Autodesk Inventor part; units mm, degrees
ref_plane "YZ Plane" through (0, 0, 0) normal (1, 0, 0) x (0, 1, 0)
ref_plane "XZ Plane" through (0, 0, 0) normal (0, 1, 0) x (-1, 0, 0)
ref_plane "XY Plane" through (0, 0, 0) normal (0, 0, 1) x (1, 0, 0)
sketch "スケッチ1" plane through (0, 0, 0) normal (1, 0, 0) x (0, 1, 0)
  circle A0 centre (0, 0) radius 19.5
  dimension "d0" = 39
extrude "押し出し1" add sketch "スケッチ1" along normal blind 3
sketch "スケッチ2" plane through (0, 0, 0) normal (-1, 0, 0) x (0, 0, 1)
  circle A0 centre (0, 0) radius 11
  point P0 (0, 11)
  point P1 (-7.7782, 7.7782)
  point P2 (-11, 0)
  point P3 (-7.7782, -7.7782)
  point P4 (0, -11)
  point P5 (7.7782, -7.7782)
  point P6 (11, 0)
  point P7 (7.7782, 7.7782)
  dimension "d3" = 22
  dimension "d6" = 360
hole "穴1" at (0, 7.7782, -7.7782) at (0, 11, 0) at (0, 7.7782, 7.7782) at (0, -7.7782, 7.7782) at (0, -11, 0) at (0, -7.7782, -7.7782) direction (1, 0, 0) diameter 2.5 end through all
sketch "スケッチ3" plane through (3, 0, 0) normal (1, 0, 0) x (0, 0, -1)
  circle A0 centre (-7.7782, 7.7782) radius 1.25
  circle A1 centre (0, 11) radius 1.25
  circle A2 centre (7.7782, 7.7782) radius 1.25
  circle A3 centre (7.7782, -7.7782) radius 1.25
  circle A4 centre (0, -11) radius 1.25
  circle A5 centre (-7.7782, -7.7782) radius 1.25
  point P0 (0, 0)
hole "穴2" [suppressed]
sketch "スケッチ4" plane through (0, 0, 0) normal (-1, 0, 0) x (0, 0, 1)
  circle A0 centre (0, 0) radius 19.5
  circle A1 centre (0, 0) radius 13
  dimension "d22" = 26
extrude "押し出し2" add sketch "スケッチ4" along normal blind 3.8 contours A1
sketch "スケッチ5" plane through (-3.8, 0, 0) normal (-1, 0, 0) x (0, 0, 1)
  point P0 (0, 0)
  point P1 (0, 11)
  point P2 (0, 11)
  point P3 (-7.7782, 7.7782)
  point P4 (-11, 0)
  point P5 (-7.7782, -7.7782)
  point P6 (0, -11)
  point P7 (7.7782, -7.7782)
  point P8 (11, 0)
  point P9 (7.7782, 7.7782)
  dimension "d27" = 360
hole "穴3" at (-3.8, 11, 0) at (-3.8, 7.7782, -7.7782) at (-3.8, 7.7782, 7.7782) at (-3.8, -7.7782, 7.7782) at (-3.8, -11, 0) at (-3.8, -7.7782, -7.7782) direction (1, 0, 0) diameter 2.5 end through all
sketch "スケッチ6" plane through (-3.8, 0, 0) normal (-1, 0, 0) x (0, 0, 1)
  circle A0 centre (0, 0) radius 5.5
  dimension "d36" = 11
extrude "押し出し3" cut sketch "スケッチ6" against normal blind 10
properties part number "connectplate5" material "アルミニウム 6061"
Part model, mm, in its own coordinate system. A direction names the side the tool comes from. Coordinates: 2 decimals unless noted, no trailing zeros. Write each loop counter-clockwise with the first axis right and the second up, starting at its lowest first coordinate (ties: lowest second). Pieces come first, ordered by that corner, then holes. Notation, with made-up numbers: M -8,62 L 29,62 A16 ccw 29,84 Z; hole C 62.5,8.25 d8. An arc over 180 degrees is marked long. Return JSON: item names as keys, results as strings.
1. Saw through at B-B, the plane y = -0.5. Write the cut outline in (x, z).
Determined:
{"outline": "M -3.8,-12.99 L 0,-12.99 L 0,-19.49 L 3,-19.49 L 3,-5.48 L -3.8,-5.48 Z; M -3.8,5.48 L 3,5.48 L 3,19.49 L 0,19.49 L 0,12.99 L -3.8,12.99 Z"}
2. Saw through at D-D, the plane z = -8. Write the cut outline in (x, y).
Determined:
{"outline": "M -3.8,-10.25 L 0,-10.25 L 0,-17.78 L 3,-17.78 L 3,-9.01 L -3.8,-9.01 Z; M -3.8,-6.55 L 3,-6.55 L 3,6.55 L -3.8,6.55 Z; M -3.8,9.01 L 3,9.01 L 3,17.78 L 0,17.78 L 0,10.25 L -3.8,10.25 Z"}
3. Saw through at C-C, the plane x = -1.5. Write the cut outline in (y, z).
Determined:
{"outline": "C 0,0 d26; hole C -11,0 d2.5; hole C -7.78,-7.78 d2.5; hole C -7.78,7.78 d2.5; hole C 0,0 d11; hole C 7.78,-7.78 d2.5; hole C 7.78,7.78 d2.5; hole C 11,0 d2.5"}
4. Saw through at A-A, the plane z = 0. Write the cut outline in (x, y).
Determined:
{"outline": "M -3.8,-13 L 0,-13 L 0,-19.5 L 3,-19.5 L 3,-12.25 L -3.8,-12.25 Z; M -3.8,-9.75 L 3,-9.75 L 3,-5.5 L -3.8,-5.5 Z; M -3.8,5.5 L 3,5.5 L 3,9.75 L -3.8,9.75 Z; M -3.8,12.25 L 3,12.25 L 3,19.5 L 0,19.5 L 0,13 L -3.8,13 Z"}
5. Pull direction Z, two halves, no side cores. Call faces 3 (the face through (-0.45, -5.37, -1.19)), 4 (the face through (3, 4, -4)), 5 (the face through (1.479, -2.539, -19.334)), 6 (the face through (-0.35, -12.24, -0.16)): pulls with the +Z half, pulls with the -Z half, needs draft (parallel to the pull), parting line crosses it, or undercut.
Determined:
{"face 3": "undercut", "face 4": "needs draft", "face 5": "parting line crosses it", "face 6": "undercut"}
6. 3-axis set-ups, long thin cutter, end or side, ignore diameter. For faces 1 (the face through (-0.352, -7.299, -6.624)), 2 (the face through (0, 4, -13)): which of +Z, -Z, +X, -X, +Y, -Y reach the whole face in a straight line?
Determined:
{"face 1": "+X, -X", "face 2": "-X"}
7. Flat gauge pins, fed straight in: pin 1 Ø1 at (x, z) = (0, 10.5) entering from +Y; pin 2 Ø3 at (x, y) = (1, -2) entering from +Z. Where does each tip first touch, or does it go through?
Determined:
{"pin 1": "y = 16.74", "pin 2": "z = 19.49"}
8. Probe L1, parallel to Y at x = -1, z = 0; L2, parallel to X at y = -5, z = -18; L3, parallel to Z at x = -2, y = 5. List the from-to ranges inside material, lowest first.
Determined:
{"L1": "-13 to -12.25, -9.75 to -5.5, 5.5 to 9.75, 12.25 to 13", "L2": "0 to 3", "L3": "-12 to -2.29, 2.29 to 12"}
